Geometry check sheet. Reference: the model listing, model coordinates, mm. A direction names the side the tool comes from. Round coordinates to 2 decimals unless told otherwise and drop trailing zeros. Write each loop counter-clockwise with the first axis right and the second up, starting at its lowest first coordinate (ties: lowest second). Pieces come first, ordered by that corner, then holes. Notation, with made-up numbers: (-19.5, 76) -> (22.5, 76) arc R12 ccw to (22.5, 88) -> close; hole circle Ø7 at (15.25, -9). An arc over 180 degrees is marked (long way). Return JSON: item names as keys, results as strings. Group by question number.
from build123d import *

# Parameters (mm, degrees)
CUT_EXTRUDE1_DEPTH      = 31.298514815
CUT_EXTRUDE1_DEPTH_BACK = 31.298514815
SKETCH2_W               = 2
SKETCH2_H               = 1.2


with BuildPart() as part:
    # Sketch1 → Revolve1 (revolve)
    with BuildSketch(Plane.XY, mode=Mode.PRIVATE) as revolve1_sk:
        Polygon((4, 3), (4, 1.8), (7, 1.8), (7, 3), (30, 3), (30, 0), (0, 0), (0, 3), align=None)
    revolve(revolve1_sk.sketch.rotate(Axis((0, 0, 0), (1, 0, 0)), 90), axis=Axis((0, 0, 0), (1, 0, 0)))

    # Sketch2 → Cut-Extrude1 (cut, two sides: drawn at the far end of the back side and taken through both)
    with BuildSketch(Plane.XY.offset(-CUT_EXTRUDE1_DEPTH_BACK)):
        with Locations((1, 0)):
            Rectangle(SKETCH2_W, SKETCH2_H)
    extrude(amount=CUT_EXTRUDE1_DEPTH + CUT_EXTRUDE1_DEPTH_BACK, mode=Mode.SUBTRACT)


solid = part.part
1) Sectioned sample at D-D on x = 22.75. Enter the section's corners in (y, z), and give its area (3 significant figures).
2) Sectioned sample at B-B on z = 0. Enter the section's corners in (x, y), and give its area (3 significant figures).
3) Sectioned sample at A-A on y = 2.65. Enter the section's corners in (x, z), and give its area (3 significant figures).
4) Sectioned sample at C-C on y = 0. Enter the section's corners in (x, z).
5) Go/stop test with flat-tipped pins: P1, Ø2, axis at x = 20, z = -1.5, coming from the +Y side; P2, Ø1.6, axis at x = 1.5, z = -1, coming from the -Y side; P3, Ø1.5, axis at x = 9.5, y = 1, coming from the -Z side. Record where each tip stops, or that it passes through.
6) Material ranges on probe 1 along X at (y, z) = (2.3, 0.1); probe 2 along X at (y, z) = (-0.45, -1.85); probe 3 along Z at (x, y) = (10.25, -0.2), recorded low to high. Write a range as [from, to].
7) Tool access check on faces 4 (the face through (1, 0.6, 0)), 5 (the face through (4, 2, 0)), 6 (the face through (18.66, -0.9, 2.86)). Record the directions out of +Z, -Z, +X, -X, +Y, -Y that give a thin tool (end or side, any length) a straight path to the whole face; none if there is none.
8) Mould release check, pull along Y, two halves, no side actions. Record for faces 1 (the face through (0, 2, 0)), 2 (the face through (1, -0.6, 0)), 3 (the face through (2.03, -0.9, 2.86)): +Y half, -Y half, draft (parallel to the pull), parting line (faces both ways), or undercut.
Evaluation:
{
 "1": {"outline": "circle Ø6 at (0, 0)", "area": "28.3 mm2"},
 "2": {"outline": "(0, -3) -> (4, -3) -> (4, -1.8) -> (7, -1.8) -> (7, -3) -> (30, -3) -> (30, 3) -> (7, 3) -> (7, 1.8) -> (4, 1.8) -> (4, 3) -> (0, 3) -> (0, 0.6) -> (2, 0.6) -> (2, -0.6) -> (0, -0.6) -> close", "area": "170 mm2"},
 "3": {"outline": "(0, -1.41) -> (4, -1.41) -> (4, 1.41) -> (0, 1.41) -> close; (7, -1.41) -> (30, -1.41) -> (30, 1.41) -> (7, 1.41) -> close", "area": "75.9 mm2"},
 "4": {"outline": "(2, -3) -> (4, -3) -> (4, -1.8) -> (7, -1.8) -> (7, -3) -> (30, -3) -> (30, 3) -> (7, 3) -> (7, 1.8) -> (4, 1.8) -> (4, 3) -> (2, 3) -> close"},
 "5": {"P1": "stops at y = 2.96", "P2": "stops at y = -2.99", "P3": "stops at z = -2.99"},
 "6": {"probe 1": "x = [0, 4], [7, 30]", "probe 2": "x = [2, 4], [7, 30]", "probe 3": "z = [-2.99, 2.99]"},
 "7": {"face 4": "+Z, -Z, -X", "face 5": "none", "face 6": "+X, -X"},
 "8": {"face 1": "draft", "face 2": "undercut", "face 3": "parting line"}
}
